```python
from build123d import *

# Parameters (mm, degrees)
F1_DEPTH = 40
F2_R     = 4.15
F2_R_2   = 3.1
F3_DEPTH = 55.001
F4_R     = 0.5
F2_R_3   = 7.25
F5_DEPTH = 6
F2_R_4   = 5.5
F6_DEPTH = 9


with BuildPart() as f1:
    # F0 (on Front) → F1 (new body)
    with BuildSketch(Plane.XZ):
        Polygon((35, 21), (-20, 21), (-20, 0), (-4.1, 0), (-4.1, -4), (4.1, -4), (4.1, 0), (20, 0), (20, -35), (35, -35), align=None)
    extrude(amount=F1_DEPTH)

    # F2 (on face) → F3 (cut, through all)
    with BuildSketch(Plane.YZ.offset(35)):
        with Locations((-20, -20)):
            Circle(F2_R)
        with Locations((-20, 5.1)):
            Circle(F2_R_2)
    extrude(amount=-F3_DEPTH, mode=Mode.SUBTRACT)

    # F4
    f4_edges = [f1.edges().sort_by_distance(p)[0] for p in [
        (-20, -20, 0),
        (-4.1, -20, -4),
        (4.1, -20, -4),
        (20, -20, 0),
        (20, -20, -35),
        (35, -20, -35),
    ]]
    fillet(f4_edges, radius=F4_R)

    # F2 (on face) → F5 (cut)
    with BuildSketch(Plane.YZ.offset(35)):
        with Locations((-20, -20)):
            Circle(F2_R_3)
        with Locations((-20, -20)):
            Circle(F2_R, mode=Mode.SUBTRACT)
    extrude(amount=-F5_DEPTH, mode=Mode.SUBTRACT)

    # F2 (on face) → F6 (cut)
    with BuildSketch(Plane.YZ.offset(35)):
        with Locations((-20, 5.1)):
            Circle(F2_R_4)
        with Locations((-20, 5.1)):
            Circle(F2_R_2, mode=Mode.SUBTRACT)
    extrude(amount=-F6_DEPTH, mode=Mode.SUBTRACT)


solid = f1.part
```
Build history of the part. All positions in model axes, mm. A direction names the side the tool comes from. Round coordinates to 2 decimals unless told otherwise and drop trailing zeros. Write each loop counter-clockwise with the first axis right and the second up, starting at its lowest first coordinate (ties: lowest second). Pieces come first, ordered by that corner, then holes. Notation, with made-up numbers: (77, 33) -> (129, 33) arc R24 cw to (129, 56) -> close; hole circle Ø5 at (42, 58.5). An arc over 180 degrees is marked (long way). Put each result on its own line as item: value.
Item 1: Slice it at B-B, the plane z = -1.5. Give the cut face in (x, y), plus the area to 3 significant figures.
Here are the results:
outline: (-4.1, -40) -> (4.1, -40) -> (4.1, 0) -> (-4.1, 0) -> close; (20, -40) -> (35, -40) -> (35, 0) -> (20, 0) -> close
area: 928 mm^2
Item 2: Two-plate mould, pull along Z, no slides. Class faces 1 (the face through (-20, -20, 11)), 2 (the face through (-12, -20, 0)), 3 (the face through (26, -17.6, 2.7)): pulls with the +Z half, pulls with the -Z half, needs draft (parallel to the pull), parting line crosses it, or undercut.
Here are the results:
face 1: needs draft
face 2: pulls with the -Z half
face 3: undercut
Item 3: Slice it at A-A, the plane y = -20. Count the separate pieces of the cut face and the enclosed holes in it, plus the area to 3 significant figures.
Here are the results:
separate pieces: 3
enclosed holes: 0
area: 1,170 mm^2
Item 4: Slice it at D-D, the plane y = -4. Give the cut face in (x, z), plus the area to 3 significant figures.
Here are the results:
outline: (-20, 0.5) arc R0.5 ccw to (-19.5, 0) -> (-4.1, 0) -> (-4.1, -3.5) arc R0.5 ccw to (-3.6, -4) -> (3.6, -4) arc R0.5 ccw to (4.1, -3.5) -> (4.1, 0) -> (19.5, 0) arc R0.5 cw to (20, -0.5) -> (20, -34.5) arc R0.5 ccw to (20.5, -35) -> (34.5, -35) arc R0.5 ccw to (35, -34.5) -> (35, 21) -> (-20, 21) -> close
area: 1,710 mm^2
Item 5: Tool access for faces 4 (the face through (4.1, -20, -2)), 5 (the face through (32.042, -25.344, -15.1)), 6 (the face through (27, -20, -35)), 7 (the face through (35, -20, -7)), 8 (the face through (-4.1, -20, -2)): list every direction of +Z, -Z, +X, -X, +Y, -Y with a clear straight run to the whole face (end or side of a thin tool).
Here are the results:
face 4: -Z, +Y, -Y
face 5: +X
face 6: -Z, +X, -X, +Y, -Y
face 7: +Z, -Z, +X, +Y, -Y
face 8: -Z, -X, +Y, -Y
Item 6: Slice it at C-C, the plane x = -2.5. Give the cut face in (y, z), plus the area to 3 significant figures.
Here are the results:
outline: (-40, -4) -> (0, -4) -> (0, 21) -> (-40, 21) -> close; hole circle Ø6.2 at (-20, 5.1)
area: 970 mm^2
Item 7: Wall check: probe 1 along Z at (x, y) = (27, -20); probe 2 along Z at (x, y) = (31.25, -20); probe 3 along Z at (x, y) = (16, -20). Give the ranges that are in metal, low to high. Write a range as from..to.
Here are the results:
probe 1: z = -35..-24.15, -15.85..-0.4, 10.6..21
probe 2: z = -35..-27.25, -12.75..-0.4, 10.6..21
probe 3: z = 0..2, 8.2..21
Item 8: Flat gauge pins, fed straight in: P1, Ø9.5, axis at y = -20, z = -20, coming from the +X side; P2, Ø7.5, axis at x = 15.5, y = -22, coming from the -Z side; P3, Ø10, axis at y = -12.5, z = -17, coming from the -X side. Where does each tip first touch, or does it go through?
Here are the results:
P1: stops at x = 29
P2: stops at z = 0
P3: stops at x = 20
